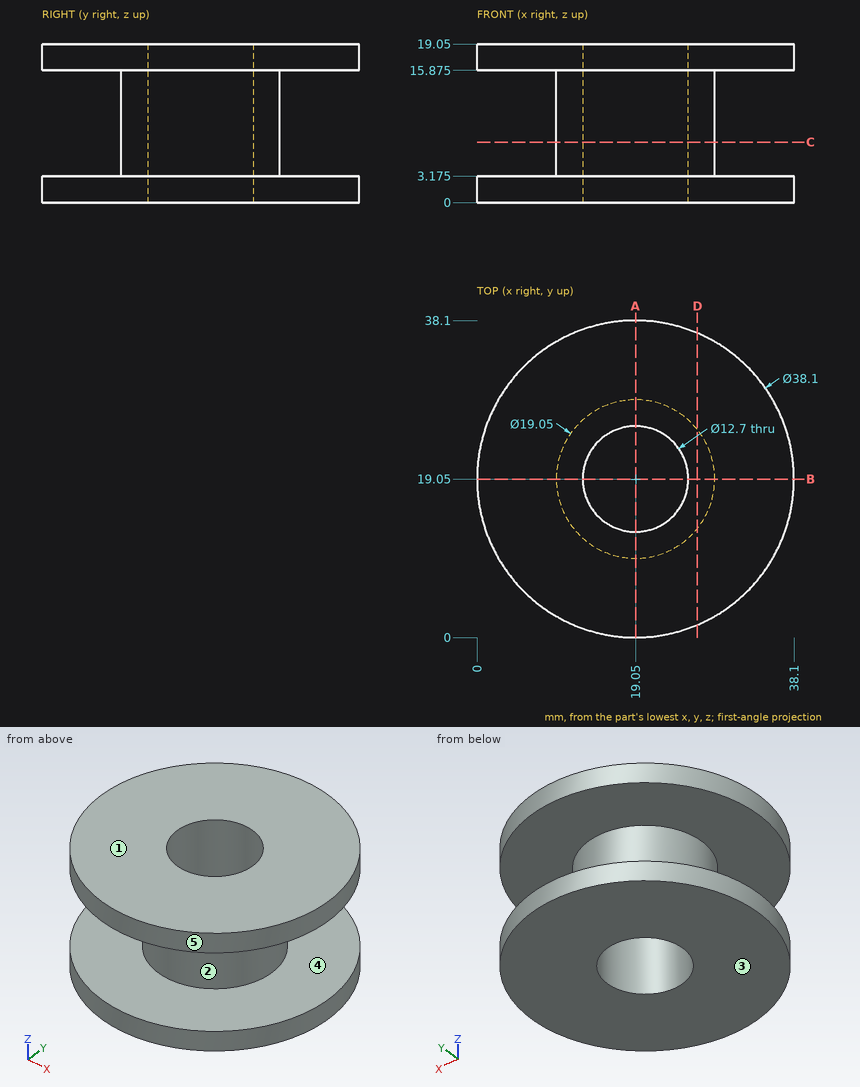
Study the drawing (mm; zero at the part's minimum x, y, z) and answer. A direction names the side the tool comes from. Give positions to 0.01 mm unless a question says otherwise; leave off trailing zeros. Write each loop counter-clockwise with the first axis right and the second up, starting at its lowest first coordinate (ties: lowest second). Pieces come first, ordered by that corner, then holes.
(1) The mould has two halves that part along Z. Classify the marked faces 1, 2 and 3: pulls with the +Z half, pulls with the -Z half, needs draft (parallel to the pull), parting line crosses it, or undercut.
Final values:
face 1: pulls with the +Z half
face 2: undercut
face 3: pulls with the -Z half
(2) Which of the six approach directions +Z, -Z, +X, -X, +Y, -Y give full straight-line access (tool end or side, diameter ignored) to the marked faces 4 and 5?
Final values:
face 4: none
face 5: +Z, -Z
(3) Straight lines are drawn through the part: line 1 (Z direction, x = 34, y = 8.5) (3 decimals); line 2 (Y direction, x = 19.05, z = 9.5) (3 decimals); line 3 (Y direction, x = 20.5, z = 6.5). For each, find the intervals that lie inside material, in ascending order.
Final values:
line 1: z = 0 to 3.175, 15.875 to 19.05
line 2: y = 9.525 to 12.7, 25.4 to 28.575
line 3: y = 9.64 to 12.87, 25.23 to 28.46
(4) The part is cut by section D-D on x = 26.5. Write down the section's boundary in (y, z) (3 decimals), plus the area to 3 significant figures.
Final values:
outline: (1.517, 0) - (36.583, 0) - (36.583, 3.175) - (24.985, 3.175) - (24.985, 15.875) - (36.583, 15.875) - (36.583, 19.05) - (1.517, 19.05) - (1.517, 15.875) - (13.115, 15.875) - (13.115, 3.175) - (1.517, 3.175) - close
area: 373 mm2
(5) Flat-ended cylindrical pins translate along their axes: pin 1 Ø10 at (y, z) = (15, 10) entering from -X (3 decimals); pin 2 Ø3 at (x, z) = (25, 12) entering from +Y; pin 3 Ø5 at (x, z) = (17.5, 8) entering from -Y (3 decimals). Find the tip coordinate at first contact, or state that the pin passes through.
Final values:
pin 1: stops at x = 9.525
pin 2: stops at y = 27.47
pin 3: stops at y = 9.525
(6) The part is cut by section C-C on z = 7.25. Write down the section's boundary in (x, y) (3 decimals).
Final values:
outline: circle Ø19.05 at (19.05, 19.05); hole circle Ø12.7 at (19.05, 19.05)
(7) The part is cut by section A-A on x = 19.05. Write down the section's boundary in (y, z) (3 decimals).
Final values:
outline: (0, 0) - (12.7, 0) - (12.7, 19.05) - (0, 19.05) - (0, 15.875) - (9.525, 15.875) - (9.525, 3.175) - (0, 3.175) - close; (25.4, 0) - (38.1, 0) - (38.1, 3.175) - (28.575, 3.175) - (28.575, 15.875) - (38.1, 15.875) - (38.1, 19.05) - (25.4, 19.05) - close
